Input: part model. Units: mm. Frame: model coordinates. Coordinates: 2 decimals unless noted, no trailing zeros. Write each loop counter-clockwise with the first axis right and the second up, starting at its lowest first coordinate (ties: lowest second). Pieces come first, ordered by that corner, then holes.
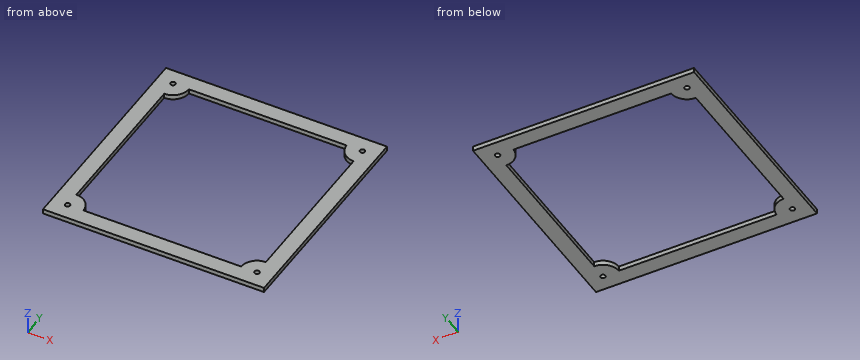
from build123d import *

# Parameters (mm, degrees)
SKETCH_1_W          = 140
SKETCH_1_H          = 140
SKETCH_1_R          = 1.55
EXTRUDE_1_DEPTH     = 3
CUT_EXTRUDE_1_DEPTH = 100.040395799


with BuildPart() as part:
    # 草圖1 → 填料-伸長1 (new body)
    with BuildSketch(Plane.XY):
        Rectangle(SKETCH_1_W, SKETCH_1_H)
        with Locations((-60, 60)):
            Circle(SKETCH_1_R, mode=Mode.SUBTRACT)
        with Locations((60, 60)):
            Circle(SKETCH_1_R, mode=Mode.SUBTRACT)
        with Locations((60, -60)):
            Circle(SKETCH_1_R, mode=Mode.SUBTRACT)
        with Locations((-60, -60)):
            Circle(SKETCH_1_R, mode=Mode.SUBTRACT)
    extrude(amount=EXTRUDE_1_DEPTH)

    # 草圖2 → 除料-伸長1 (cut, through all)
    with BuildSketch(Plane.XY.offset(3)):
        with BuildLine():
            Line((-50, -60), (50, -60))
            ThreePointArc((50, -60), (52.928932188, -52.928932188), (60, -50))
            Line((60, -50), (60, 50))
            ThreePointArc((60, 50), (52.928932188, 52.928932188), (50, 60))
            Line((50, 60), (-50, 60))
            ThreePointArc((-50, 60), (-52.928932188, 52.928932188), (-60, 50))
            Line((-60, 50), (-60, -50))
            ThreePointArc((-60, -50), (-52.928932188, -52.928932188), (-50, -60))
        make_face()
    extrude(amount=-CUT_EXTRUDE_1_DEPTH, mode=Mode.SUBTRACT)


solid = part.part
Item 1: Section query C-C, the plane z = 1.5. Return loops of the section in (x, y).
Item 2: Section query A-A, the plane y = -41. Return loops of the section in (x, z).
Item 3: Material intervals for line 1 (Y direction, x = 48, z = 1.6); line 2 (X direction, y = -58, z = 0.4), sorted ascending.
The answers:
1. outline: (-70, -70) - (70, -70) - (70, 70) - (-70, 70) - close; hole circle Ø3.1 at (-60, -60); hole circle Ø3.1 at (-60, 60); hole (-60, -50) arc R10 cw to (-50, -60) - (50, -60) arc R10 cw to (60, -50) - (60, 50) arc R10 cw to (50, 60) - (-50, 60) arc R10 cw to (-60, 50) - close; hole circle Ø3.1 at (60, -60); hole circle Ø3.1 at (60, 60)
2. outline: (-70, 0) - (-60, 0) - (-60, 3) - (-70, 3) - close; (60, 0) - (70, 0) - (70, 3) - (60, 3) - close
3. line 1: y = -70 to -60, 60 to 70
3. line 2: x = -70 to -50.2, 50.2 to 70
